Drawing for the job (mm, zero at the part's lowest x, y, z). A direction names the side the tool comes from. Give positions to 0.01 mm unless a question says otherwise; leave off trailing zeros. Loops run counter-clockwise (first coordinate to the right, second up) from the corner with the lowest first, then second, coordinate; pieces in that order, holes last. Notation, with made-up numbers: (-33.5, 20.5) -> (-6.5, 20.5) arc R19 ccw to (-6.5, 56.5) -> close; hole circle Ø4 at (55.25, -26). An arc over 180 degrees is marked (long way). Write item = value, one per line.
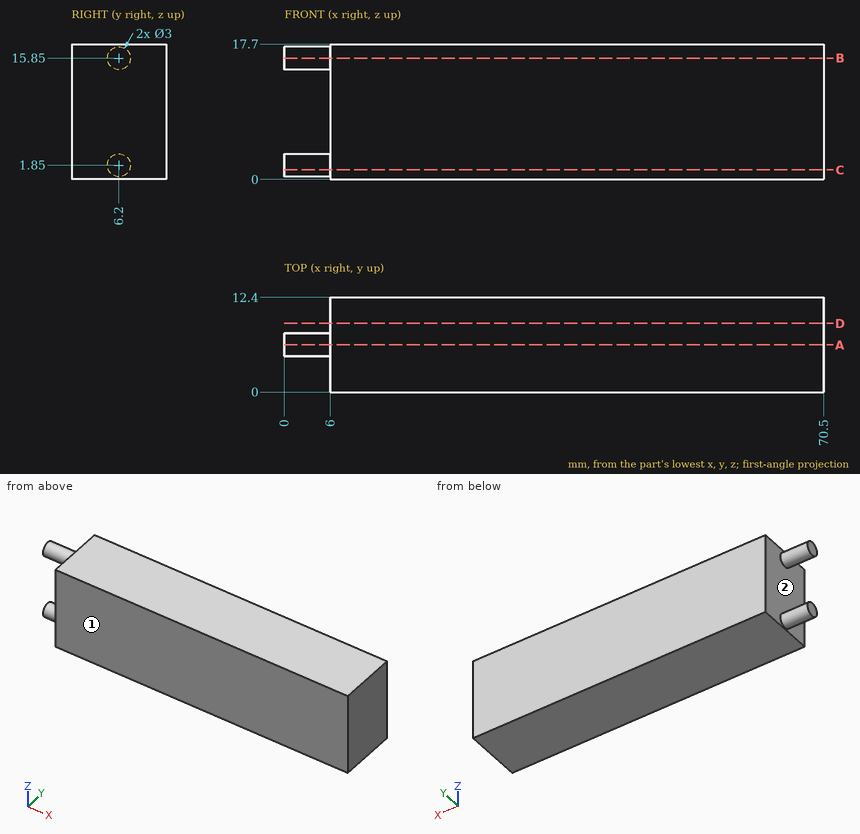
1) Which spindle directions (+Z, -Z, +X, -X, +Y, -Y) get a long thin tool onto all of the face, cutting with end or side? Do the marked faces 1 and 2. Say none if no direction does.
Resolved:
face_1 = +Z, -Z, +X, -X, -Y
face_2 = -X
2) Drill centre line: line 1 along X through (y, z) = (2.5, 7.25). Where is it in solid material? Low to high. Write a range as [from, to].
Resolved:
line_1 = [6, 70.5]
3) Slice it at A-A, the plane y = 6.2. List the corners of the cut face in (x, z), and give its area (3 significant figures).
Resolved:
outline = (0, 0.35) -> (6, 0.35) -> (6, 0) -> (70.5, 0) -> (70.5, 17.7) -> (6, 17.7) -> (6, 17.35) -> (0, 17.35) -> (0, 14.35) -> (6, 14.35) -> (6, 3.35) -> (0, 3.35) -> close
area = 1,180 mm²
4) Slice it at D-D, the plane y = 9. List the corners of the cut face in (x, z).
Resolved:
outline = (6, 0) -> (70.5, 0) -> (70.5, 17.7) -> (6, 17.7) -> close
5) Slice it at C-C, the plane z = 1.25. List the corners of the cut face in (x, y).
Resolved:
outline = (0, 4.83) -> (6, 4.83) -> (6, 0) -> (70.5, 0) -> (70.5, 12.4) -> (6, 12.4) -> (6, 7.57) -> (0, 7.57) -> close
6) Drop a flat-ended pin along its axis: P1, Ø1.5, axis at y = 6.5, z = 13, coming from the -X side. Give the stop position or say it passes through.
Resolved:
P1 = 6
7) Slice it at B-B, the plane z = 15.85. List the corners of the cut face in (x, y).
Resolved:
outline = (0, 4.7) -> (6, 4.7) -> (6, 0) -> (70.5, 0) -> (70.5, 12.4) -> (6, 12.4) -> (6, 7.7) -> (0, 7.7) -> close
